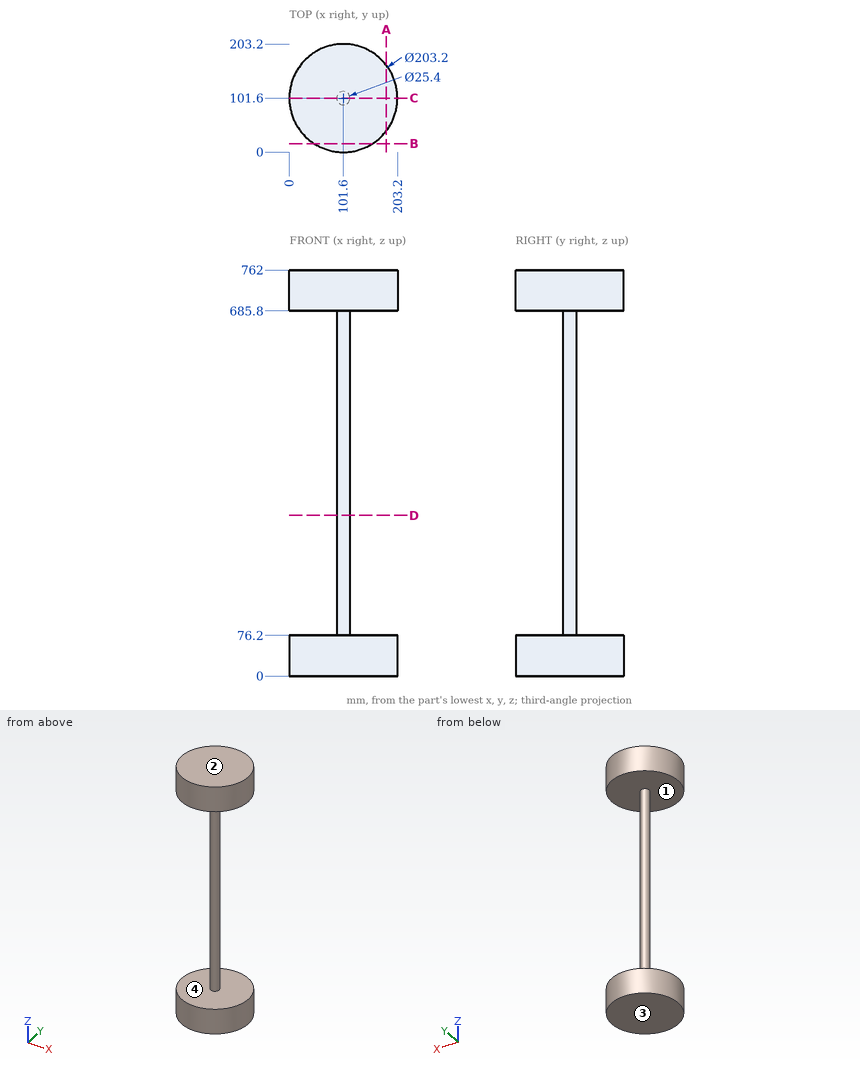
Geometry: see drawing. Coordinates: mm, zero at the bounding-box minimum. Give positions to 0.01 mm unless a question says otherwise; leave off trailing zeros. Write each loop counter-clockwise with the first axis right and the second up, starting at its lowest first coordinate (ties: lowest second). Pieces come first, ordered by that corner, then holes. Notation, with made-up numbers: M -21,-14.5 L -12,-14.5 A4 ccw -12,-8.5 Z; hole C 10.5,-31 d1. An arc over 180 degrees is marked long. Answer in a Markdown table with one row per item. Add a question column.
(1) Section B-B on y = 16. Return loops of the section in (x, z), and give its area (3 significant figures).
(2) Ray query, line 1 (Z direction, x = 157, y = 162.5); line 2 (X direction, y = 101.5, z = 182.5); line 3 (X direction, y = 105, z = 695). Return the intervals inside material, ascending.
(3) Mould query, pull axis Z, two halves, no side actions, for the marked faces 1, 2, 3 and 4. Classes: +Z half, -Z half, draft (parallel to the pull), parting line (faces both ways), or undercut.
(4) First-contact query: pin 1 (10 mm diameter, centred on y = 113.5, z = 420.5, fed in from +X); pin 2 (12 mm diameter, centred on y = 24, z = 81.5, fed in from -X). Flat tips, straight axial feed; report the tip coordinate or a pass-through.
(5) Section D-D on z = 301.5. Return loops of the section in (x, y), and give its area (3 significant figures).
(6) Section A-A on x = 182.5. Return loops of the section in (y, z).
(7) Section C-C on y = 101.6. Return loops of the section in (x, z), and give its area (3 significant figures).
Result set:
| question | item | result |
|---|---|---|
| 1 | outline | M 46.87,0 L 156.33,0 L 156.33,76.2 L 46.87,76.2 Z; M 46.87,685.8 L 156.33,685.8 L 156.33,762 L 46.87,762 Z |
| 1 | area | 16,700 mm^2 |
| 2 | line 1 | z = 0 to 76.2, 685.8 to 762 |
| 2 | line 2 | x = 88.9 to 114.3 |
| 2 | line 3 | x = 0.06 to 203.14 |
| 3 | face 1 | undercut |
| 3 | face 2 | +Z half |
| 3 | face 3 | -Z half |
| 3 | face 4 | undercut |
| 4 | pin 1 | stops at x = 112.26 |
| 4 | pin 2 | stops at x = 32.83 |
| 5 | outline | C 101.6,101.6 d25.4 |
| 5 | area | 507 mm^2 |
| 6 | outline | M 40.14,0 L 163.06,0 L 163.06,76.2 L 40.14,76.2 Z; M 40.14,685.8 L 163.06,685.8 L 163.06,762 L 40.14,762 Z |
| 7 | outline | M 0,0 L 203.2,0 L 203.2,76.2 L 114.3,76.2 L 114.3,685.8 L 203.2,685.8 L 203.2,762 L 0,762 L 0,685.8 L 88.9,685.8 L 88.9,76.2 L 0,76.2 Z |
| 7 | area | 46,500 mm^2 |
